Work out the finished part from the listing and answer in its coordinate system (mm). A direction names the side the tool comes from. Round coordinates to 2 decimals unless told otherwise and drop trailing zeros. Order: outer loops, then holes, each group sorted by start corner. A loop starts at its lowest first (then second) coordinate and runs counter-clockwise, first axis right, second up. Notation, with made-up numbers: (65.5, 11.5) -> (100.5, 11.5) arc R15 cw to (100.5, 38.5) -> close; hole circle Ø2 at (-30.5, 23). An arc over 180 degrees is marked (long way). Use a Markdown table: item, result. Add a question column.
Item 1: A cutting plane is placed at C-C, the plane z = 10.25. Determine the outline of the cut face in (x, y).
Item 2: For a pull along Y with two mould halves and no side action, classify faces 3 (the cylindrical face through (-7.493, -0.33, 11.678)), 4 (the conical face through (3.75, -1.18, -2.09)), 5 (the flat face through (-2, 1, -9.238)) as +Y half, -Y half, draft (parallel to the pull), parting line (faces both ways), or undercut.
Item 3: Flat-ended cylindrical pins translate along their axes: P1, Ø2, axis at y = 4, z = -5, coming from the -X side; P2, Ø5, axis at x = -3, z = 5.5, coming from the -Y side; P3, Ø8, axis at y = -4.5, z = 1.5, coming from the +X side. Find the tip coordinate at first contact, or state that the pin passes through.
Item 4: A cutting plane is placed at D-D, the plane z = 3.25. Determine the outline of the cut face in (x, y).
Item 5: A cutting plane is placed at A-A, the plane x = 0. Determine the outline of the cut face in (y, z) (3 decimals).
Item 6: A tool of negligible diameter and unlimited length cuts with its end or side. For faces 1 (the flat face through (4, -4, 17.762)), 2 (the cylindrical face through (-1.19, 5.37, 11.85)), from which of +Z, -Z, +X, -X, +Y, -Y can it reach the whole face along a straight path? Write none if from no direction.
Item 7: Find the intervals of material crossed by L1, parallel to Y at x = 0, z = 12.5; L2, parallel to X at y = -2, z = -5.75, in increasing order. Write a range as [from, to].
from build123d import *

# Parameters (mm, degrees)
CHAMFER1_SIZE  = 0.5
CHAMFER1_SIZE2 = 0.637377439


with BuildPart() as part:
    # Sketch1 → Revolve1 (revolve)
    with BuildSketch(Plane(origin=(0, 0, 0), x_dir=(1, 0, 0), z_dir=(0, 1, 0))):
        Polygon((2, 9.237606838), (2, 7.237606838), (2.9, 7.237606838), (5.5, -5.762393162), (5.5, -17.762393162), (7.5, -17.762393162), (7.5, -5.762393162), (4.5, 9.237606838), align=None)
    revolve(axis=Axis((0, 0, 0), (0, 0, -1)))

    # Chamfer1
    chamfer1_edges = [part.edges().sort_by_distance(p)[0] for p in [
        (-4.5, 0, -9.237606838),
    ]]
    chamfer1_side = [part.faces().sort_by_distance(p)[0] for p in [
        (-4.372720779, 0, -9.237606838),
    ]]
    chamfer(chamfer1_edges, length=CHAMFER1_SIZE, length2=CHAMFER1_SIZE2, reference=chamfer1_side[0])


solid = part.part
Reported:
| question | item | result |
|---|---|---|
| 1 | outline | circle Ø15 at (0, 0); hole circle Ø11 at (0, 0) |
| 2 | face 3 | parting line |
| 2 | face 4 | undercut |
| 2 | face 5 | draft |
| 3 | P1 | x = -4.47 |
| 3 | P2 | y = -7.48 |
| 3 | P3 | x = 7.02 |
| 4 | outline | circle Ø14 at (0, 0); hole circle Ø10 at (0, 0) |
| 5 | outline | (-7.5, 5.762) -> (-4.625, -8.613) -> (-4, -9.238) -> (-2, -9.238) -> (-2, -7.238) -> (-2.9, -7.238) -> (-5.5, 5.762) -> (-5.5, 17.762) -> (-7.5, 17.762) -> close; (2, -9.238) -> (4, -9.238) -> (4.625, -8.613) -> (7.5, 5.762) -> (7.5, 17.762) -> (5.5, 17.762) -> (5.5, 5.762) -> (2.9, -7.238) -> (2, -7.238) -> close |
| 6 | face 1 | +Z, +X, -X, +Y, -Y |
| 6 | face 2 | +Z |
| 7 | L1 | [-7.5, -5.5], [5.5, 7.5] |
| 7 | L2 | [-4.8, -2.49], [2.49, 4.8] |
